Source: CAD feature listing. Evaluate the final solid. Frame: model axes, mm. A direction names the side the tool comes from. Coordinates: 2 decimals unless noted, no trailing zeros. Loops run counter-clockwise (first coordinate to the right, second up) from the corner with the lowest first, then second, coordinate; pieces in that order, holes last. Notation, with made-up numbers: (61, -37.5) -> (69, -37.5) arc R29 cw to (69, -10.5) -> close; hole circle Ø6 at (87.25, 13.25). An arc over 180 degrees is marked (long way). Answer as CSV lines item,"result".
from build123d import *

# Parameters (mm, degrees)
SKETCH1_R           = 3.175
SKETCH1_R_2         = 0.8
SKETCH1_R_3         = 1.5
SKETCH1_W           = 6.35
SKETCH1_H           = 12.7
BOSS_EXTRUDE1_DEPTH = 3.175
CUT_EXTRUDE1_DEPTH  = 7.35
CUT_EXTRUDE2_DEPTH  = 7.35


with BuildPart() as part:
    # Sketch1 → Boss-Extrude1 (new body, symmetric)
    with BuildSketch(Plane.XY):
        with BuildLine():
            Line((52.705, 9.525), (52.705, -9.525))
            Line((52.705, -9.525), (1.260352874, -23.642702569))
            ThreePointArc((1.260352874, -23.642702569), (0.451437295, -23.791055855), (-0.370940015, -23.798032198))
            Line((-0.370940015, -23.798032198), (-61.330940015, -19.035532198))
            ThreePointArc((-61.330940015, -19.035532198), (-65.616640497, -15.286051717), (-63.245106279, -10.109019948))
            Line((-63.245106279, -10.109019948), (-2.285106279, 23.228480052))
            ThreePointArc((-2.285106279, 23.228480052), (-0.552652656, 23.780325707), (1.260352874, 23.642702569))
            Line((1.260352874, 23.642702569), (52.705, 9.525))
        make_face()
        Circle(SKETCH1_R, mode=Mode.SUBTRACT)
        with Locations((-3.889087297, 3.889087297)):
            Circle(SKETCH1_R_2, mode=Mode.SUBTRACT)
        with Locations((3.889087297, -3.889087297)):
            Circle(SKETCH1_R_2, mode=Mode.SUBTRACT)
        with Locations((30.48, 0)):
            Circle(SKETCH1_R_3, mode=Mode.SUBTRACT)
        with Locations((-30.48, 0)):
            Circle(SKETCH1_R_3, mode=Mode.SUBTRACT)
        with Locations((3.889087297, 3.889087297)):
            Circle(SKETCH1_R_2, mode=Mode.SUBTRACT)
        with Locations((-3.889087297, -3.889087297)):
            Circle(SKETCH1_R_2, mode=Mode.SUBTRACT)
        with Locations((0, -19.05)):
            Circle(SKETCH1_R_3, mode=Mode.SUBTRACT)
        with Locations((0, 19.05)):
            Circle(SKETCH1_R_3, mode=Mode.SUBTRACT)
        with Locations((46.355, 0)):
            Rectangle(SKETCH1_W, SKETCH1_H, mode=Mode.SUBTRACT)
    extrude(amount=BOSS_EXTRUDE1_DEPTH, both=True)

    # Sketch2 → Cut-Extrude1 (cut, through all)
    with BuildSketch(Plane.XY.offset(3.175)):
        with BuildLine():
            Line((-6.334889923, -16.962749429), (-54.842346338, -13.173104397))
            Line((-54.842346338, -13.173104397), (-33.871837797, -3.343178518))
            ThreePointArc((-33.871837797, -3.343178518), (-30.766203139, -4.753892512), (-27.513752337, -3.72596042))
            Line((-27.513752337, -3.72596042), (-6.334889923, -16.962749429))
        make_face()
        with BuildLine():
            Line((25.7175, 11.992472423), (25.7175, -11.992472423))
            Line((25.7175, -11.992472423), (6.049537699, -17.389854996))
            ThreePointArc((6.049537699, -17.389854996), (9.525, 0), (6.049537699, 17.389854996))
            Line((6.049537699, 17.389854996), (25.7175, 11.992472423))
        make_face()
    extrude(amount=-CUT_EXTRUDE1_DEPTH, mode=Mode.SUBTRACT)

    # Sketch3 → Cut-Extrude2 (cut, through all)
    with BuildSketch(Plane.XY.offset(3.175)):
        with BuildLine():
            Line((-1.5875, -16.185756869), (-24.944710991, -1.5875))
            Line((-24.944710991, -1.5875), (-9.391776656, -1.5875))
            ThreePointArc((-9.391776656, -1.5875), (-6.735192091, -6.735192091), (-1.5875, -9.391776656))
            Line((-1.5875, -9.391776656), (-1.5875, -16.185756869))
        make_face()
    cut_extrude2 = extrude(amount=-CUT_EXTRUDE2_DEPTH, mode=Mode.SUBTRACT)

    # Mirror1: Cut-Extrude2 across plane
    add(cut_extrude2.mirror(Plane.ZX), mode=Mode.SUBTRACT)


solid = part.part
(1) Pin query (flat end, axial travel): pin 1 Ø1.9 at (x, z) = (-17, 0) entering from +Y; pin 2 Ø2 at (x, z) = (9, 2) entering from +Y; pin 3 Ø1 at (x, z) = (-8, -0.5) entering from +Y. Return the tip coordinate at first contact, or that it passes through.
Computed values:
pin 1,"y = 15.7"
pin 2,"y = 21.79"
pin 3,"y = 20.38"
(2) Cut plane D-D (x = 30.48). Return the cut outline in (y, z) (3 decimals).
Computed values:
outline,"(-15.624, -3.175) -> (-1.5, -3.175) -> (-1.5, 3.175) -> (-15.624, 3.175) -> close; (1.5, -3.175) -> (15.624, -3.175) -> (15.624, 3.175) -> (1.5, 3.175) -> close"
(3) Access query for faces 1 (the flat face through (-30.2, -15.1, 0)), 2 (the flat face through (26.623, 16.683, 0.044)). Directions: +Z, -Z, +X, -X, +Y, -Y. A direction counts if a zero-diameter tool reaches every point of the face in a straight line with its end or side. Return the directions, or none.
Computed values:
face 1,"+Z, -Z"
face 2,"+Z, -Z, +X, +Y"
(4) Material intervals for L1, parallel to X at y = 5.5, z = 3 (1 decimal); L2, parallel to Y at x = -21.5, z = -1.75; L3, parallel to X at y = 4.5, z = 1.25 (1 decimal), sorted ascending. Write a range as [from, to].
Computed values:
L1,"[-34.7, -18.7], [-7.8, 9.2], [25.7, 43.2], [49.5, 52.7]"
L2,"[-22.15, -15.78], [-7.48, -3.74], [-1.59, 1.59], [3.74, 12.72]"
L3,"[-36.5, -20.3], [-8.4, -4.4], [-3.4, 3.4], [4.4, 9.3], [25.7, 43.2], [49.5, 52.7]"
(5) Cut plane B-B (y = 0). Return the cut outline in (x, z) (1 decimal).
Computed values:
outline,"(-44.8, -3.2) -> (-32, -3.2) -> (-32, 3.2) -> (-44.8, 3.2) -> close; (-29, -3.2) -> (-3.2, -3.2) -> (-3.2, 3.2) -> (-29, 3.2) -> close; (3.2, -3.2) -> (9.5, -3.2) -> (9.5, 3.2) -> (3.2, 3.2) -> close; (25.7, -3.2) -> (29, -3.2) -> (29, 3.2) -> (25.7, 3.2) -> close; (32, -3.2) -> (43.2, -3.2) -> (43.2, 3.2) -> (32, 3.2) -> close; (49.5, -3.2) -> (52.7, -3.2) -> (52.7, 3.2) -> (49.5, 3.2) -> close"
(6) Cut plane A-A (x = -12). Return the cut outline in (y, z) (1 decimal), then the cut area to 3 significant figures.
Computed values:
outline,"(-22.9, -3.2) -> (-16.5, -3.2) -> (-16.5, 3.2) -> (-22.9, 3.2) -> close; (-13.4, -3.2) -> (-9.7, -3.2) -> (-9.7, 3.2) -> (-13.4, 3.2) -> close; (-1.6, -3.2) -> (1.6, -3.2) -> (1.6, 3.2) -> (-1.6, 3.2) -> close; (9.7, -3.2) -> (17.9, -3.2) -> (17.9, 3.2) -> (9.7, 3.2) -> close"
area,"137 mm^2"
(7) Cut plane C-C (y = 19.05). Return the cut outline in (x, z) (3 decimals), then the cut area to 3 significant figures.
Computed values:
outline,"(-9.926, -3.175) -> (-1.5, -3.175) -> (-1.5, 3.175) -> (-9.926, 3.175) -> close; (1.5, -3.175) -> (17.996, -3.175) -> (17.996, 3.175) -> (1.5, 3.175) -> close"
area,"158 mm^2"
(8) Draft query along X for faces 3 (the flat face through (27.343, -16.485, 0.044)), 4 (the cylindrical face through (9.524, -0.25, 0.044)), 5 (the flat face through (-30.42, -21.45, 0.04)). Return one class per face: released by +X, released by -X, zero draft, split by the parting line, or undercut.
Computed values:
face 3,"released by +X"
face 4,"undercut"
face 5,"released by -X"
